```python
from build123d import *

# Parameters (mm, degrees)
SKETCH1_R                    = 55.88
SKETCH1_R_2                  = 46.99
BOSS_EXTRUDE4_DEPTH          = 101.6
SKETCH3_R                    = 50.8
CUT_EXTRUDE3_DEPTH           = 1.5875
F_1_4_28_TAPPED_HOLE1_REACH  = 156.393
F_1_4_28_TAPPED_HOLE1_BORE_R = 2.7051


with BuildPart() as part:
    # Sketch1 → Boss-Extrude4 (new body)
    with BuildSketch(Plane(origin=(0, 0, 0), x_dir=(1, 0, 0), z_dir=(0, 1, 0))):
        with Locations(Location((0, 0, 0), (0, 0, 270))):
            Circle(SKETCH1_R)
        with Locations(Location((0, 0, 0), (0, 0, 270))):
            Circle(SKETCH1_R_2, mode=Mode.SUBTRACT)
    extrude(amount=-BOSS_EXTRUDE4_DEPTH)

    # Sketch3 → Cut-Extrude3 (cut)
    with BuildSketch(Plane(origin=(0, 0, 0), x_dir=(1, 0, 0), z_dir=(0, 1, 0))):
        with Locations(Location((0, 0, 0), (0, 0, 270))):
            Circle(SKETCH3_R)
    extrude(amount=-CUT_EXTRUDE3_DEPTH, mode=Mode.SUBTRACT)

    # 1/4-28 Tapped Hole1 bore (on position points) → 1/4-28 Tapped Hole1 (cut, up to next)
    with BuildSketch(Plane(origin=(-54.781474323, -84.349985228, 11.025627917), x_dir=(-0.197309017847, 0, -0.980341344368), z_dir=(-0.980341344368, 0, 0.197309017847)), mode=Mode.PRIVATE) as f_1_4_28_tapped_hole1_sk1:
        Circle(F_1_4_28_TAPPED_HOLE1_BORE_R)
    f_1_4_28_tapped_hole1_tool1 = extrude(f_1_4_28_tapped_hole1_sk1.sketch, amount=-F_1_4_28_TAPPED_HOLE1_REACH, mode=Mode.PRIVATE) & part.part
    add(f_1_4_28_tapped_hole1_tool1.solids().sort_by_distance((-54.781474, -84.349985, 11.025628))[0], mode=Mode.SUBTRACT)


solid = part.part
```
Geometry check sheet. Reference: the model listing, model coordinates, mm. A direction names the side the tool comes from. Round coordinates to 2 decimals unless told otherwise and drop trailing zeros. Order: outer loops, then holes, each group sorted by start corner. A loop starts at its lowest first (then second) coordinate and runs counter-clockwise, first axis right, second up. Notation, with made-up numbers: (68.25, 52) - (99.25, 52) arc R29 cw to (99.25, 83) - close; hole circle Ø11 at (21.5, 88.25). An arc over 180 degrees is marked (long way). Use a Markdown table: item, result. Add a question column.
(1) Sectioned sample at C-C, the plane y = -37. Enter the section's corners in (x, z), and give its area (3 significant figures).
(2) Sectioned sample at D-D, the plane z = -48.5. Enter the section's corners in (x, y), and give its area (3 significant figures).
(3) Sectioned sample at B-B, the plane x = 0. Enter the section's corners in (y, z).
(4) Depth check by flat-ended pin: pin 1 (10 mm diameter, centred on x = -42, y = -38, fed in from -Z); pin 2 (2 mm diameter, centred on y = -85, z = -35.5, fed in from -X); pin 3 (2 mm diameter, centred on x = 35.5, y = -28.5, fed in from +Z). Enter the tip coordinate at first touch or a pass-through.
(5) Sectioned sample at A-A, the plane z = 0. Enter the section's corners in (x, y), and give its area (3 significant figures).
(6) Release check for a two-part mould opening along Z. For faces 1 (the flat face through (-49.4, 0, -12.7)), 2 (the cylindrical face through (55.4, -50.1, -7.3)), 3 (the cylindrical face through (-45.87, -50.89, -10.19)) record: pulls with the +Z half, pulls with the -Z half, needs draft (parallel to the pull), parting line crosses it, or undercut.
(7) Tool access check on faces 4 (the cylindrical face through (-50.33, -81.71, 10.73)), 5 (the flat face through (-45, -1.588, 15)). Record the directions out of +Z, -Z, +X, -X, +Y, -Y that give a thin tool (end or side, any length) a straight path to the whole face; none if there is none.
(8) Material ranges on line 1 along X through (y, z) = (-1.05, 0); line 2 along X through (y, z) = (-51.5, 0); line 3 along Y through (x, z) = (-48, 12), recorded low to high. Write a range as [from, to].
Answers below:
| question | item | result |
|---|---|---|
| 1 | outline | circle Ø111.76 at (0, 0); hole circle Ø93.98 at (0, 0) |
| 1 | area | 2,870 mm² |
| 2 | outline | (-27.75, -101.6) - (27.75, -101.6) - (27.75, 0) - (15.11, 0) - (15.11, -1.59) - (-15.11, -1.59) - (-15.11, 0) - (-27.75, 0) - close |
| 2 | area | 5,590 mm² |
| 3 | outline | (-101.6, -55.88) - (0, -55.88) - (0, -50.8) - (-1.59, -50.8) - (-1.59, -46.99) - (-101.6, -46.99) - close; (-101.6, 46.99) - (-1.59, 46.99) - (-1.59, 50.8) - (0, 50.8) - (0, 55.88) - (-101.6, 55.88) - close |
| 4 | pin 1 | z = -41.88 |
| 4 | pin 2 | x = -43.96 |
| 4 | pin 3 | z = 43.96 |
| 5 | outline | (-55.88, -101.6) - (-46.99, -101.6) - (-46.99, -1.59) - (-50.8, -1.59) - (-50.8, 0) - (-55.88, 0) - close; (46.99, -101.6) - (55.88, -101.6) - (55.88, 0) - (50.8, 0) - (50.8, -1.59) - (46.99, -1.59) - close |
| 5 | area | 1,790 mm² |
| 6 | face 1 | needs draft |
| 6 | face 2 | parting line crosses it |
| 6 | face 3 | undercut |
| 7 | face 4 | none |
| 7 | face 5 | +Y |
| 8 | line 1 | [-55.88, -50.8], [50.8, 55.88] |
| 8 | line 2 | [-55.88, -46.99], [46.99, 55.88] |
| 8 | line 3 | [-101.6, -85.78], [-82.92, -1.59] |
